```python
from build123d import *

# Parameters (mm, degrees)
SKETCH1_W           = 22
SKETCH1_H           = 64
BOSS_EXTRUDE2_DEPTH = 49
SKETCH3_W           = 18.5
SKETCH3_H           = 64
CUT_EXTRUDE1_DEPTH  = 20
SKETCH4_R           = 2.14
CUT_EXTRUDE2_DEPTH  = 28
SKETCH5_W           = 64
SKETCH5_H           = 6
BOSS_EXTRUDE3_DEPTH = 18.5
SKETCH6_W           = 2.4
SKETCH6_H           = 64
BOSS_EXTRUDE4_DEPTH = 19
SKETCH7_R           = 3.41
CUT_EXTRUDE3_DEPTH  = 13
SKETCH8_W           = 64
SKETCH8_H           = 6
BOSS_EXTRUDE5_DEPTH = 18.5
SKETCH9_W           = 2.4
SKETCH9_H           = 64
BOSS_EXTRUDE6_DEPTH = 19
SKETCH10_R          = 3.41
CUT_EXTRUDE4_DEPTH  = 13.550505831
SKETCH12_R          = 3.075953135
CUT_EXTRUDE6_DEPTH  = 50
CUT_EXTRUDE7_REACH  = 42.5
SKETCH13_W          = 31.75
SKETCH13_H          = 6
SKETCH15_W          = 2.4
SKETCH15_H          = 43.25
CUT_EXTRUDE8_DEPTH  = 19
SKETCH16_W          = 2.4
SKETCH16_H          = 43.25
CUT_EXTRUDE9_DEPTH  = 19
SKETCH17_R          = 3.075953135
SKETCH17_W          = 18.5
SKETCH17_H          = 11.5
CUT_EXTRUDE10_DEPTH = 3.6


with BuildPart() as part:
    # Sketch1 → Boss-Extrude2 (new body)
    with BuildSketch(Plane(origin=(0, 0, 0), x_dir=(1, 0, 0), z_dir=(0, 1, 0))):
        Rectangle(SKETCH1_W, SKETCH1_H)
    extrude(amount=BOSS_EXTRUDE2_DEPTH)

    # Sketch3 → Cut-Extrude1 (cut)
    with BuildSketch(Plane(origin=(0, 49, 0), x_dir=(1, 0, 0), z_dir=(0, 1, 0))):
        Rectangle(SKETCH3_W, SKETCH3_H)
    extrude(amount=-CUT_EXTRUDE1_DEPTH, mode=Mode.SUBTRACT)

    # Sketch4 → Cut-Extrude2 (cut)
    with BuildSketch(Plane(origin=(11, 0, 0), x_dir=(0, 0, -1), z_dir=(1, 0, 0))):
        with Locations((20.979041052, 37.382)):
            Circle(SKETCH4_R)
    extrude(amount=-CUT_EXTRUDE2_DEPTH, mode=Mode.SUBTRACT)

    # Sketch5 → Boss-Extrude3 (add)
    with BuildSketch(Plane(origin=(11, 0, 0), x_dir=(0, 0, -1), z_dir=(1, 0, 0))):
        with Locations((0, 3)):
            Rectangle(SKETCH5_W, SKETCH5_H)
    extrude(amount=BOSS_EXTRUDE3_DEPTH)

    # Sketch6 → Boss-Extrude4 (add)
    with BuildSketch(Plane(origin=(0, 6, 0), x_dir=(1, 0, 0), z_dir=(0, 1, 0))):
        with Locations((28.3, 0)):
            Rectangle(SKETCH6_W, SKETCH6_H)
    extrude(amount=BOSS_EXTRUDE4_DEPTH)

    # Sketch7 → Cut-Extrude3 (cut)
    with BuildSketch(Plane(origin=(29.5, 0, 0), x_dir=(0, 0, -1), z_dir=(1, 0, 0))):
        with Locations((21, 12.5)):
            Circle(SKETCH7_R)
    extrude(amount=-CUT_EXTRUDE3_DEPTH, mode=Mode.SUBTRACT)

    # Sketch8 → Boss-Extrude5 (add)
    with BuildSketch(Plane.ZY.offset(11)):
        with Locations((0, 3)):
            Rectangle(SKETCH8_W, SKETCH8_H)
    extrude(amount=BOSS_EXTRUDE5_DEPTH)

    # Sketch9 → Boss-Extrude6 (add)
    with BuildSketch(Plane(origin=(0, 6, 0), x_dir=(1, 0, 0), z_dir=(0, 1, 0))):
        with Locations((-28.3, 0)):
            Rectangle(SKETCH9_W, SKETCH9_H)
    extrude(amount=BOSS_EXTRUDE6_DEPTH)

    # Sketch10 → Cut-Extrude4 (cut)
    with BuildSketch(Plane.ZY.offset(29.5)):
        with Locations((-21, 12.5)):
            Circle(SKETCH10_R)
    extrude(amount=-CUT_EXTRUDE4_DEPTH, mode=Mode.SUBTRACT)

    # Sketch12 → Cut-Extrude6 (cut, through all)
    with BuildSketch(Plane(origin=(0, 0, 0), x_dir=(-1, 0, 0), z_dir=(0, -1, 0))):
        with Locations((14.6918, -4.628600023)):
            Circle(SKETCH12_R)
        with Locations((-14.6918, -4.628600023)):
            Circle(SKETCH12_R)
    extrude(amount=-CUT_EXTRUDE6_DEPTH, mode=Mode.SUBTRACT)

    # Sketch13 → Cut-Extrude7 (cut, up to next)
    with BuildSketch(Plane.ZY.offset(11), mode=Mode.PRIVATE) as cut_extrude7_sk1:
        with Locations((4.625, 9)):
            Rectangle(SKETCH13_W, SKETCH13_H)
    cut_extrude7_tool1 = extrude(cut_extrude7_sk1.sketch, amount=-CUT_EXTRUDE7_REACH, mode=Mode.PRIVATE) & part.part
    add(cut_extrude7_tool1.solids().sort_by_distance((-11, 9, 4.625))[0], mode=Mode.SUBTRACT)

    # Sketch15 → Cut-Extrude8 (cut)
    with BuildSketch(Plane(origin=(0, 25, 0), x_dir=(1, 0, 0), z_dir=(0, 1, 0))):
        with Locations((-28.3, -10.375)):
            Rectangle(SKETCH15_W, SKETCH15_H)
    extrude(amount=-CUT_EXTRUDE8_DEPTH, mode=Mode.SUBTRACT)

    # Sketch16 → Cut-Extrude9 (cut)
    with BuildSketch(Plane(origin=(0, 25, 0), x_dir=(1, 0, 0), z_dir=(0, 1, 0))):
        with Locations((28.3, -10.375)):
            Rectangle(SKETCH16_W, SKETCH16_H)
    extrude(amount=-CUT_EXTRUDE9_DEPTH, mode=Mode.SUBTRACT)

    # Sketch17 → Cut-Extrude10 (cut)
    with BuildSketch(Plane(origin=(0, 6, 0), x_dir=(1, 0, 0), z_dir=(0, 1, 0))):
        Polygon((-27.1, 11.25), (-29.5, 11.25), (-29.5, -20.5), (-11, -20.5), (11, -20.5), (29.5, -20.5), (29.5, 11.25), (27.1, 11.25), (11, 11.25), (-11, 11.25), align=None)
        with Locations((-14.6918, -4.628600023)):
            Circle(SKETCH17_R, mode=Mode.SUBTRACT)
        with Locations((14.6918, -4.628600023)):
            Circle(SKETCH17_R, mode=Mode.SUBTRACT)
        with Locations((-20.25, -26.25)):
            Rectangle(SKETCH17_W, SKETCH17_H)
        with Locations((20.25, -26.25)):
            Rectangle(SKETCH17_W, SKETCH17_H)
    extrude(amount=-CUT_EXTRUDE10_DEPTH, mode=Mode.SUBTRACT)


solid = part.part
```
CAD build for the part. Positions are in the model's coordinates, mm. A direction names the side the tool comes from. Round coordinates to 2 decimals unless told otherwise and drop trailing zeros. Write each loop counter-clockwise with the first axis right and the second up, starting at its lowest first coordinate (ties: lowest second). Pieces come first, ordered by that corner, then holes. Notation, with made-up numbers: M -8.75,75 L 3.25,75 A16 cw 3.25,95 Z; hole C 40.25,81.5 d7. An arc over 180 degrees is marked long. One line per question, with ' | ' between items.
1. Cut at A-A on y = 32.5. Write the cut outline in (x, z), and give its area (3 significant figures).
Working result:
outline: M -11,-32 L -9.25,-32 L -9.25,32 L -11,32 Z; M 9.25,-32 L 11,-32 L 11,32 L 9.25,32 Z | area: 224 mm2
2. Which spindle directions (+Z, -Z, +X, -X, +Y, -Y) get a long thin tool onto all of the face, cutting with end or side? Do faces 1 (the cylindrical face through (-28.317, 13.524, -17.747)), 2 (the flat face through (27.1, 17, -21)), 3 (the flat face through (0, 12, 4)). Say none if no direction does.
Working result:
face 1: -X | face 2: +Z, -Z, +Y | face 3: +X, -X
3. Pin check, flat tips, straight feed: pin 1 Ø3.5 at (x, z) = (14.69, 4.63) entering from -Y; pin 2 Ø4 at (y, z) = (36.5, -2) entering from +X; pin 3 Ø23.5 at (y, z) = (18, 13.5) entering from -X; pin 4 Ø1 at (x, z) = (3.5, 25.5) entering from +Y. Stop position of each tip, or through.
Working result:
pin 1: through | pin 2: x = 11 | pin 3: x = -11 | pin 4: y = 29
4. Probe L1, parallel to X at y = 36, z = 15.5; L2, parallel to X at y = 6.5, z = -27; L3, parallel to Y at x = -8, z = 6. List the from-to ranges inside material, lowest first. Write a range as from..to.
Working result:
L1: -11..-9.25, 9.25..11 | L2: -29.5..-27.1, -11..11, 27.1..29.5 | L3: 0..2.4, 12..29
5. Cut at D-D on x = -14. Write the cut outline in (y, z).
Working result:
outline: M 0,-32 L 6,-32 L 6,-11.25 L 2.4,-11.25 L 2.4,1.63 L 0,1.63 Z; M 0,7.63 L 2.4,7.63 L 2.4,32 L 0,32 Z
6. Mould opens along X. For faces 4 (the flat face through (-19, 6, -22)), 5 (the flat face through (0, 9, -11.25)), 6 (the flat face through (29.5, 10, -14)) say: pulls with the +X half, pulls with the -X half, needs draft (parallel to the pull), parting line crosses it, or undercut.
Working result:
face 4: undercut | face 5: needs draft | face 6: pulls with the +X half
7. Cut at B-B on x = 2. Write the cut outline in (y, z), and give its area (3 significant figures).
Working result:
outline: M 0,-32 L 29,-32 L 29,32 L 0,32 Z; hole M 2.4,-11.25 L 12,-11.25 L 12,20.5 L 2.4,20.5 Z | area: 1,550 mm2
8. Cut at C-C on z = -26.5. Write the cut outline in (x, y), and give its area (3 significant figures).
Working result:
outline: M -29.5,0 L 29.5,0 L 29.5,25 L 27.1,25 L 27.1,6 L 11,6 L 11,49 L 9.25,49 L 9.25,29 L -9.25,29 L -9.25,49 L -11,49 L -11,6 L -27.1,6 L -27.1,25 L -29.5,25 Z | area: 1,020 mm2
